from build123d import *

# Parameters (mm, degrees)
SKETCH1_R           = 7.5
BOSS_EXTRUDE1_DEPTH = 4.74
BOSS_EXTRUDE2_DEPTH = 0.74
BOSS_EXTRUDE3_START = -4
SKETCH1_4_R         = 7.5
BOSS_EXTRUDE3_DEPTH = 4
BOSS_EXTRUDE4_START = 4.74
SKETCH2_R           = 5
BOSS_EXTRUDE4_DEPTH = 4.74
BOSS_EXTRUDE5_START = 0.74
SKETCH2_3_R         = 5.5
SKETCH2_3_R_2       = 5
BOSS_EXTRUDE5_DEPTH = 0.74
SKETCH2_5_R         = 5.5
SKETCH2_5_R_2       = 5
BOSS_EXTRUDE6_DEPTH = 15.48
SKETCH2_6_R         = 5
BOSS_EXTRUDE7_DEPTH = 19.48


with BuildPart() as part:
    # Sketch1 → Boss-Extrude1 (new body)
    with BuildSketch(Plane(origin=(0, 0, 0), x_dir=(1, 0, 0), z_dir=(0, 1, 0))):
        with Locations(Location((-1, 0, 0), (0, 0, 270))):
            Circle(SKETCH1_R)
        with BuildLine():
            Line((-1.5, 2), (1.5, 2))
            ThreePointArc((1.5, 2), (0, -2.5), (-1.5, 2))
        make_face(mode=Mode.SUBTRACT)
    extrude(amount=BOSS_EXTRUDE1_DEPTH)

    # Sketch1_3 → Boss-Extrude2 (add)
    with BuildSketch(Plane(origin=(0, 0, 0), x_dir=(1, 0, 0), z_dir=(0, 1, 0))):
        with BuildLine():
            ThreePointArc((0, -7.433034374), (5.937104415, -5.645794895), (8.5, 0))
            ThreePointArc((8.5, 0), (5.937104415, 5.645794895), (0, 7.433034374))
            ThreePointArc((0, 7.433034374), (4.645794895, 4.937104415), (6.5, 0))
            ThreePointArc((6.5, 0), (4.645794895, -4.937104415), (0, -7.433034374))
        make_face()
    extrude(amount=BOSS_EXTRUDE2_DEPTH)

    # Sketch1_4 → Boss-Extrude3 (add)
    with BuildSketch(Plane(origin=(0, 0, 0), x_dir=(1, 0, 0), z_dir=(0, 1, 0)).offset(BOSS_EXTRUDE3_START)):
        with Locations(Location((1, 0, 0), (0, 0, 97.662255661))):
            Circle(SKETCH1_4_R)
        with BuildLine():
            Line((-1.5, 2), (1.5, 2))
            ThreePointArc((1.5, 2), (0, -2.5), (-1.5, 2))
        make_face(mode=Mode.SUBTRACT)
    extrude(amount=BOSS_EXTRUDE3_DEPTH)

    # Sketch2 → Boss-Extrude4 (add)
    with BuildSketch(Plane.XZ.offset(4).offset(BOSS_EXTRUDE4_START)):
        with Locations(Location((0, 0, 0), (0, 0, 90))):
            Circle(SKETCH2_R)
        with BuildLine():
            Line((1.5, -2), (-1.5, -2))
            ThreePointArc((-1.5, -2), (0, 2.5), (1.5, -2))
        make_face(mode=Mode.SUBTRACT)
    extrude(amount=-BOSS_EXTRUDE4_DEPTH)

    # Sketch2_3 → Boss-Extrude5 (add)
    with BuildSketch(Plane.XZ.offset(4).offset(BOSS_EXTRUDE5_START)):
        with Locations(Location((0, 0, 0), (0, 0, 90))):
            Circle(SKETCH2_3_R)
        with Locations(Location((0, 0, 0), (0, 0, 270))):
            Circle(SKETCH2_3_R_2, mode=Mode.SUBTRACT)
    extrude(amount=-BOSS_EXTRUDE5_DEPTH)

    # Sketch2_5 → Boss-Extrude6 (add)
    with BuildSketch(Plane.XZ.offset(4)):
        with Locations(Location((0, 0, 0), (0, 0, 90))):
            Circle(SKETCH2_5_R)
        with Locations(Location((0, 0, 0), (0, 0, 270))):
            Circle(SKETCH2_5_R_2, mode=Mode.SUBTRACT)
    extrude(amount=-BOSS_EXTRUDE6_DEPTH)

    # Sketch2_6 → Boss-Extrude7 (add)
    with BuildSketch(Plane.XZ.offset(4)):
        with Locations(Location((0, 0, 0), (0, 0, 270))):
            Circle(SKETCH2_6_R)
        with BuildLine():
            Line((1.5, -2), (-1.5, -2))
            ThreePointArc((-1.5, -2), (0, 2.5), (1.5, -2))
        make_face(mode=Mode.SUBTRACT)
    extrude(amount=-BOSS_EXTRUDE7_DEPTH)


solid = part.part
Could you check a few things on this model? Use its own coordinates, in mm. A direction names the side the tool comes from. Coordinates: 2 decimals unless noted, no trailing zeros. Loops run counter-clockwise (first coordinate to the right, second up) from the corner with the lowest first, then second, coordinate; pieces in that order, holes last.
1. I need wall thicknesses on L1, parallel to X at y = 12.25, z = 0; L2, parallel to X at y = 9.25, z = 0; L3, parallel to Y at x = -3.25, z = -4.5. Which ranges of each line are inside material? Lowest first, please.
2. For P1, Ø5, axis at x = -2.5, y = 2.5, coming from the +Z side; P2, Ø3.5, axis at x = 0, y = -7, coming from the +Z side; P3, Ø3, axis at x = 0, z = 0, coming from the -Y side; P4, Ø0.9, axis at x = -0.5, y = 8.5, coming from the +Z side, each with a flat end and sliding along its axis, tell me the tip position at first contact or that it passes through.
3. For faces 1 (the face through (-7, 0, 0)), 2 (the face through (5.37, 8.06, -1.19)), 3 (the face through (7, 0.74, 1)), 4 (the face through (4.9, -4.74, 1.6)), 5 (the face through (-0.1, -8.74, -2.3)), which set-ups out of +Z, -Z, +X, -X, +Y, -Y let a thin tool reach every point of the face, with its end or its side?
4. Imagine slicing it at D-D (y = 9). Please give me the cut outline in (x, z), and give its area (3 significant figures).
5. Imagine slicing it at C-C (x = 3). Please give me the cut outline in (y, z).
6. Imagine slicing it at A-A (x = 1). Please give me the cut outline in (y, z), and give its area (3 significant figures).
7. Imagine slicing it at B-B (y = -5.75). Please give me the cut outline in (x, z), and give its area (3 significant figures).
Computed values:
1. L1: x = -5 to -2.5, 2.5 to 5
1. L2: x = -5.5 to -2.5, 2.5 to 5.5
1. L3: y = -4 to 4.74
2. P1: stops at z = 7.5
2. P2: stops at z = 5
2. P3: passes through
2. P4: stops at z = 5.5
3. face 1: -X, -Y
3. face 2: +Y
3. face 3: +X, +Y
3. face 4: -Y
3. face 5: +Z, -Z, +X, -X, -Y
4. outline: circle Ø11 at (0, 0); hole (-1.5, -2) - (1.5, -2) arc R2.5 ccw (long way) to start
4. area: 76.4 mm2
5. outline: (-8.74, -4) - (-4.74, -4) - (-4.74, -4.61) - (-4, -4.61) - (-4, -7.23) - (0.74, -7.23) - (0.74, -6.34) - (4.74, -6.34) - (4.74, -4.61) - (11.48, -4.61) - (11.48, -4) - (15.48, -4) - (15.48, 4) - (11.48, 4) - (11.48, 4.61) - (4.74, 4.61) - (4.74, 6.34) - (0.74, 6.34) - (0.74, 7.23) - (-4, 7.23) - (-4, 4.61) - (-4.74, 4.61) - (-4.74, 4) - (-8.74, 4) - close
6. outline: (-8.74, -4.9) - (-4.74, -4.9) - (-4.74, -5.41) - (-4, -5.41) - (-4, -7.5) - (0.74, -7.5) - (0.74, -7.23) - (4.74, -7.23) - (4.74, -5.41) - (11.48, -5.41) - (11.48, -4.9) - (15.48, -4.9) - (15.48, -2) - (-8.74, -2) - close; (-8.74, 2.29) - (15.48, 2.29) - (15.48, 4.9) - (11.48, 4.9) - (11.48, 5.41) - (4.74, 5.41) - (4.74, 7.23) - (0.74, 7.23) - (0.74, 7.5) - (-4, 7.5) - (-4, 5.41) - (-4.74, 5.41) - (-4.74, 4.9) - (-8.74, 4.9) - close
6. area: 184 mm2
7. outline: circle Ø10 at (0, 0); hole (-1.5, -2) - (1.5, -2) arc R2.5 ccw (long way) to start
7. area: 59.9 mm2
